Here's how the part is built. I have some questions about the finished solid (model axes, mm). A direction names the side the tool comes from. Round coordinates to 2 decimals unless told otherwise and drop trailing zeros. Order: outer loops, then holes, each group sorted by start corner. A loop starts at its lowest first (then second) coordinate and runs counter-clockwise, first axis right, second up. Notation, with made-up numbers: (89, 65) -> (119, 65) arc R9 ccw to (119, 74) -> close; hole circle Ø11 at (82, -5). An arc over 180 degrees is marked (long way). Use a Markdown table: item, result. Add a question column.
(1) If I drill on probe 1 along X at (y, z) = (4.5, 3); probe 2 along Y at (x, z) = (-33.5, 2.5); probe 3 along Y at (x, z) = (-38.5, 5.5), over which ranges is the centre line in solid material (lowest first)?
(2) Thinking about a two-plate mould opening in X: for faces 5 (the face through (-47.98, -1.39, 2.52)), 6 (the face through (-20.655, -1.419, 2.521)), 7 (the face through (-35, 1.861, 5)), which applies, pulls with the +X half, pulls with the -X half, needs draft (parallel to the pull), parting line crosses it, or undercut?
(3) I want a section at C-C, the plane y = 5.75. Please give me the cut outline in (x, z).
(4) I want a section at A-A, the plane z = 1.75. Give the number of separate pieces and of enclosed holes in the cut face, then the cut area to 3 significant figures.
(5) I'm going to push flat-ended pins straight in: P1, Ø2, axis at y = 5.5, z = 6.5, coming from the -X side; P2, Ø2.5, axis at x = -38, z = 5.5, coming from the +Y side; P3, Ø0.6, axis at x = -34.5, z = 5, coming from the +Y side. Where does each tip first touch, or does it pass through?
(6) On a 3-axis mill with a long thin cutter (end or side, diameter ignored), from which of +Z, -Z, +X, -X, +Y, -Y can I reach the whole of each face in a straight line? I mean faces 1 (the face through (-21.424, 11.11, 2.521)), 2 (the face through (-48.253, 5.335, 0.285)), 3 (the face through (-38, 3.761, 7)), 4 (the face through (-31, 3.761, 7)). Say none if no direction works.
(7) I want a section at D-D, the plane x = -30.25. Please give me the cut outline in (y, z).
from build123d import *

# Parameters (mm, degrees)
CROQUIS1_W              = 28.5
CROQUIS1_H              = 14.5
SALIENTE_EXTRUIR1_DEPTH = 1
CROQUIS2_W              = 28.5
CROQUIS2_H              = 14.5
CROQUIS2_W_2            = 26.9
CROQUIS2_H_2            = 12.9
SALIENTE_EXTRUIR2_DEPTH = 3
SALIENTE_EXTRUIR3_DEPTH = 8
CORTAR_EXTRUIR1_DEPTH   = 5
SALIENTE_EXTRUIR4_DEPTH = 3
REDONDEO1_R             = 2
REDONDEO2_R             = 1


with BuildPart() as part:
    # Croquis1 → Saliente-Extruir1 (new body)
    with BuildSketch(Plane.XY):
        with Locations((-34.303237222, 5.261061947)):
            Rectangle(CROQUIS1_W, CROQUIS1_H)
    extrude(amount=SALIENTE_EXTRUIR1_DEPTH)

    # Croquis2 → Saliente-Extruir2 (add)
    with BuildSketch(Plane.XY.offset(1)):
        with Locations((-34.303237222, 5.261061947)):
            Rectangle(CROQUIS2_W, CROQUIS2_H)
        with Locations((-34.303237222, 5.261061947)):
            Rectangle(CROQUIS2_W_2, CROQUIS2_H_2, mode=Mode.SUBTRACT)
    extrude(amount=SALIENTE_EXTRUIR2_DEPTH)

    # Croquis3 → Saliente-Extruir3 (add)
    with BuildSketch(Plane.XY.offset(1)):
        Polygon((-39.203237222, 8.661061947), (-34.903237222, 8.661061947), (-34.903237222, 9.361061947), (-34.203237222, 9.361061947), (-34.203237222, 8.661061947), (-29.903237222, 8.661061947), (-29.903237222, 1.861061947), (-31.903237222, 1.861061947), (-31.903237222, 1.161061947), (-32.603237222, 1.161061947), (-32.603237222, 1.861061947), (-36.503237222, 1.861061947), (-36.503237222, 1.161061947), (-37.203237222, 1.161061947), (-37.203237222, 1.861061947), (-39.203237222, 1.861061947), align=None)
    extrude(amount=SALIENTE_EXTRUIR3_DEPTH)

    # Croquis4 → Cortar-Extruir1 (cut)
    with BuildSketch(Plane.XY.offset(9)):
        Polygon((-39.203237222, 6.761061947), (-37.021186236, 6.761061947), (-37.021186236, 5.261061947), (-37.021186236, 3.761061947), (-39.203237222, 3.761061947), (-39.203237222, 2.761061947), (-35.521186236, 2.761061947), (-35.521186236, 5.261061947), (-35.521186236, 7.761061947), (-39.203237222, 7.761061947), align=None)
        Polygon((-29.903237222, 3.761061947), (-32.085288209, 3.761061947), (-32.085288209, 5.261061947), (-32.085288209, 6.761061947), (-29.903237222, 6.761061947), (-29.903237222, 7.761061947), (-33.585288209, 7.761061947), (-33.585288209, 5.261061947), (-33.585288209, 2.761061947), (-29.903237222, 2.761061947), align=None)
    extrude(amount=-CORTAR_EXTRUIR1_DEPTH, mode=Mode.SUBTRACT)

    # Croquis5 → Saliente-Extruir4 (add)
    with BuildSketch(Plane.XZ.offset(-3.761061947)):
        Polygon((-39.203237222, 8.9), (-39.896057545, 7.7), (-39.203237222, 7.7), align=None)
        Polygon((-29.903237222, 7.7), (-29.903237222, 8.9), (-29.210416899, 7.7), align=None)
    extrude(amount=-SALIENTE_EXTRUIR4_DEPTH)

    # Redondeo1
    redondeo1_edges = [part.edges().sort_by_distance(p)[0] for p in [
        (-47.753237222, 11.711061947, 2.5),
        (-47.753237222, -1.188938053, 2.5),
        (-20.853237222, -1.188938053, 2.5),
        (-20.853237222, 11.711061947, 2.5),
        (-48.553237222, 12.511061947, 2),
        (-20.053237222, 12.511061947, 2),
        (-20.053237222, -1.988938053, 2),
        (-48.553237222, -1.988938053, 2),
    ]]
    fillet(redondeo1_edges, radius=REDONDEO1_R)

    # Redondeo2
    redondeo2_edges = [part.edges().sort_by_distance(p)[0] for p in [
        (-34.303237222, 12.511061947, 0),
        (-48.553237222, 5.261061947, 0),
        (-20.053237222, 5.261061947, 0),
        (-34.303237222, -1.988938053, 0),
        (-47.967450785, -1.403151615, 0),
        (-47.967450785, 11.925275509, 0),
        (-20.63902366, -1.403151615, 0),
        (-20.63902366, 11.925275509, 0),
    ]]
    fillet(redondeo2_edges, radius=REDONDEO2_R)


solid = part.part
Taken from the geometry:
| question | item | result |
|---|---|---|
| 1 | probe 1 | x = -48.55 to -47.75, -39.2 to -29.9, -20.85 to -20.05 |
| 1 | probe 2 | y = -1.99 to -1.19, 1.86 to 8.66, 11.71 to 12.51 |
| 1 | probe 3 | y = 1.86 to 2.76, 3.76 to 6.76, 7.76 to 8.66 |
| 2 | face 5 | pulls with the -X half |
| 2 | face 6 | pulls with the +X half |
| 2 | face 7 | undercut |
| 3 | outline | (-48.55, 1) arc R1 ccw to (-47.55, 0) -> (-21.05, 0) arc R1 ccw to (-20.05, 1) -> (-20.05, 4) -> (-20.85, 4) -> (-20.85, 1) -> (-29.9, 1) -> (-29.9, 7.7) -> (-29.21, 7.7) -> (-29.9, 8.9) -> (-29.9, 9) -> (-32.09, 9) -> (-32.09, 4) -> (-33.59, 4) -> (-33.59, 9) -> (-35.52, 9) -> (-35.52, 4) -> (-37.02, 4) -> (-37.02, 9) -> (-39.2, 9) -> (-39.2, 8.9) -> (-39.9, 7.7) -> (-39.2, 7.7) -> (-39.2, 1) -> (-47.75, 1) -> (-47.75, 4) -> (-48.55, 4) -> close |
| 4 | separate pieces | 2 |
| 4 | enclosed holes | 1 |
| 4 | area | 131 mm2 |
| 5 | P1 | stops at x = -39.2 |
| 5 | P2 | stops at y = 8.66 |
| 5 | P3 | stops at y = 9.36 |
| 6 | face 1 | +Z |
| 6 | face 2 | -Z, -X, +Y, -Y |
| 6 | face 3 | +Z, -X |
| 6 | face 4 | +Z, +X |
| 7 | outline | (-1.99, 1) arc R1 ccw to (-0.99, 0) -> (11.51, 0) arc R1 ccw to (12.51, 1) -> (12.51, 4) -> (11.71, 4) -> (11.71, 1) -> (8.66, 1) -> (8.66, 9) -> (7.76, 9) -> (7.76, 4) -> (6.76, 4) -> (6.76, 9) -> (3.76, 9) -> (3.76, 4) -> (2.76, 4) -> (2.76, 9) -> (1.86, 9) -> (1.86, 1) -> (-1.19, 1) -> (-1.19, 4) -> (-1.99, 4) -> close |
